```python
from build123d import *

# Parameters (mm, degrees)
SKETCH2_W           = 27
SKETCH2_H           = 42
BOSS_EXTRUDE1_DEPTH = 76
CUT_EXTRUDE1_DEPTH  = 28
CUT_EXTRUDE2_DEPTH  = 77
SKETCH5_W           = 25
SKETCH5_H           = 32
CUT_EXTRUDE3_DEPTH  = 28


with BuildPart() as part:
    # Sketch2 → Boss-Extrude1 (new body)
    with BuildSketch(Plane.XY):
        with Locations((13.5, 21)):
            Rectangle(SKETCH2_W, SKETCH2_H)
    extrude(amount=-BOSS_EXTRUDE1_DEPTH)

    # Sketch3 → Cut-Extrude1 (cut, through all)
    with BuildSketch(Plane.ZY):
        with BuildLine():
            Line((-56, 39.5), (-46, 39.5))
            ThreePointArc((-46, 39.5), (-43.5, 37), (-46, 34.5))
            Line((-46, 34.5), (-56, 34.5))
            ThreePointArc((-56, 34.5), (-58.5, 37), (-56, 39.5))
        make_face()
        with BuildLine():
            Line((-16, 39.5), (-6, 39.5))
            ThreePointArc((-6, 39.5), (-3.5, 37), (-6, 34.5))
            Line((-6, 34.5), (-16, 34.5))
            ThreePointArc((-16, 34.5), (-18.5, 37), (-16, 39.5))
        make_face()
        with BuildLine():
            Line((-16, 7.5), (-6, 7.5))
            ThreePointArc((-6, 7.5), (-3.5, 5), (-6, 2.5))
            Line((-6, 2.5), (-16, 2.5))
            ThreePointArc((-16, 2.5), (-18.5, 5), (-16, 7.5))
        make_face()
    extrude(amount=-CUT_EXTRUDE1_DEPTH, mode=Mode.SUBTRACT)

    # Sketch4 → Cut-Extrude2 (cut, through all)
    with BuildSketch(Plane.XY):
        with BuildLine():
            Line((11, 33), (0, 33))
            Line((0, 33), (0, 9))
            Line((0, 9), (11, 9))
            ThreePointArc((11, 9), (23, 21), (11, 33))
        make_face()
    extrude(amount=-CUT_EXTRUDE2_DEPTH, mode=Mode.SUBTRACT)

    # Sketch5 → Cut-Extrude3 (cut, through all)
    with BuildSketch(Plane(origin=(27, 0, 0), x_dir=(0, 0, -1), z_dir=(1, 0, 0))):
        with Locations((48.2, 16)):
            Rectangle(SKETCH5_W, SKETCH5_H)
    extrude(amount=-CUT_EXTRUDE3_DEPTH, mode=Mode.SUBTRACT)


solid = part.part
```
CAD build for the part. Positions are in the model's coordinates, mm. A direction names the side the tool comes from. Coordinates: 2 decimals unless noted, no trailing zeros. Order: outer loops, then holes, each group sorted by start corner. A loop starts at its lowest first (then second) coordinate and runs counter-clockwise, first axis right, second up. Notation, with made-up numbers: M 49.25,-24.5 L 107.25,-24.5 A16 ccw 107.25,-15.5 Z; hole C 69,2 d11. An arc over 180 degrees is marked long. Write each question's results on one line, items separated by ' | '. Start each with the question number.
Q1. Cut at A-A (z = -8.5). List the corners of the cut face in (x, y).
Q2. Which spindle directions (+Z, -Z, +X, -X, +Y, -Y) get a long thin tool onto all of the face, cutting with end or side? Do faces 5 (the flat face through (22.3, 26, -76)), 6 (the flat face through (17, 9, -35.7)), 7 (the flat face through (6, 33, -37)), 8 (the flat face through (13, 2.5, -11)). Say none if no direction does.
Q3. Flat gauge pins, fed straight in: P1, Ø1, axis at y = 14.5, z = -23, coming from the -X side; P2, Ø8, axis at x = 15.5, z = -51.5, coming from the -Y side; P3, Ø10, axis at x = 9.5, z = -45.5, coming from the -Y side; P4, Ø3, axis at x = 18.5, z = -7.5, coming from the -Y side. Where does each tip first touch, or does it go through?
Q4. Cut at C-C (y = 37). List the corners of the cut face in (x, z), then the cut area to 3 significant figures.
Q5. Cut at D-D (z = -51.5). List the corners of the cut face in (x, y).
Q6. Drill centre lines: probe 1 along Z at (x, y) = (6, 37); probe 2 along Y at (x, z) = (1.25, -9); probe 3 along Z at (x, y) = (7.75, 5). Where is each one in solid material? Low to high. Write a range as from..to.
Q7. Pull direction Y, two halves, no side cores. Call faces 1 (the cylindrical face through (13.3, 36.9, -58.5)), 2 (the flat face through (13, 0, -18)), 3 (the cylindrical face through (13.3, 4.9, -18.5)), 4 (the flat face through (22.3, 26, 0)): +Y half, -Y half, draft (parallel to the pull), parting line (faces both ways), or undercut.
Q8. Cut at B-B (y = 21). List the corners of the cut face in (x, z), then the cut area to 3 significant figures.
Found:
1) outline: M 0,0 L 27,0 L 27,2.5 L 0,2.5 Z; M 0,7.5 L 27,7.5 L 27,34.5 L 0,34.5 L 0,33 L 11,33 A12 cw 11,9 L 0,9 Z; M 0,39.5 L 27,39.5 L 27,42 L 0,42 Z
2) face 5: -Z, +X, -X, +Y, -Y | face 6: +X, -X, -Y | face 7: +Z, -Z, -X | face 8: +X, -X
3) P1: x = 20.75 | P2: y = 32 | P3: y = 32.48 | P4: y = 0
4) outline: M 0,-76 L 27,-76 L 27,-58.5 L 0,-58.5 Z; M 0,-43.5 L 27,-43.5 L 27,-18.5 L 0,-18.5 Z; M 0,-3.5 L 27,-3.5 L 27,0 L 0,0 Z | area: 1,240 mm²
5) outline: M 0,33 L 11,33 A12 cw 15.8,32 L 27,32 L 27,34.5 L 0,34.5 Z; M 0,39.5 L 27,39.5 L 27,42 L 0,42 Z
6) probe 1: -76..-58.5, -43.5..-18.5, -3.5..0 | probe 2: 0..2.5, 7.5..9, 33..34.5, 39.5..42 | probe 3: -76..-60.7, -35.7..-18.5, -3.5..0
7) face 1: undercut | face 2: -Y half | face 3: undercut | face 4: draft
8) outline: M 23,-76 L 27,-76 L 27,-60.7 L 23,-60.7 Z; M 23,-35.7 L 27,-35.7 L 27,0 L 23,0 Z | area: 204 mm²
